from build123d import *

# Parameters (mm, degrees)
F1_DEPTH = 6.35


with BuildPart() as f1:
    # F0 (on Front) → F1 (new body, symmetric)
    with BuildSketch(Plane.XZ):
        Polygon((0, 190.5), (-1066.8, 190.5), (-1066.8, 177.8), (-1104.9, 177.8), (-1104.9, 129.54), (-1066.8, 129.54), (-1066.8, 0), (-1066.8, -129.54), (-1104.9, -129.54), (-1104.9, -177.8), (-1066.8, -177.8), (-1066.8, -190.5), (0, -190.5), (1066.8, -190.5), (1066.8, -177.8), (1104.9, -177.8), (1104.9, -129.54), (1066.8, -129.54), (1066.8, 0), (1066.8, 129.54), (1104.9, 129.54), (1104.9, 177.8), (1066.8, 177.8), (1066.8, 190.5), align=None)
    extrude(amount=F1_DEPTH, both=True)


solid = f1.part
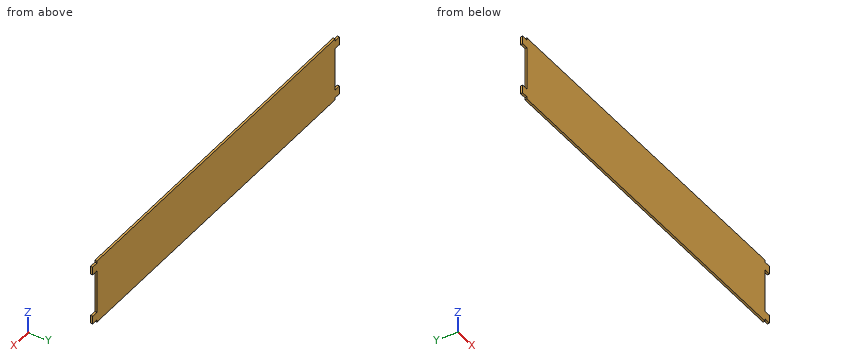
Read the model definition and answer for the solid it produces. Units are mm, in the model's axes. Give positions to 0.01 mm unless a question says otherwise; leave off trailing zeros. Loops run counter-clockwise (first coordinate to the right, second up) from the corner with the lowest first, then second, coordinate; pieces in that order, holes last. Notation, with made-up numbers: (46.25, -3.75) -> (54.25, -3.75) arc R14 cw to (54.25, 15.25) -> close; hole circle Ø7 at (65, -12). An arc over 180 degrees is marked (long way). Use a Markdown table: item, result.
Q1. Find the intervals of material crossed by line 1 along X through (y, z) = (-2.25, -79), in increasing order.
Solved:
| item | result |
|---|---|
| line 1 | x = -1066.8 to 1066.8 |
Q2. Section A-A, the plane y = 0.75 is taken. Determine the outline of the cut face in (x, z), then the cut area to 3 significant figures.
Solved:
| item | result |
|---|---|
| outline | (-1104.9, -177.8) -> (-1066.8, -177.8) -> (-1066.8, -190.5) -> (1066.8, -190.5) -> (1066.8, -177.8) -> (1104.9, -177.8) -> (1104.9, -129.54) -> (1066.8, -129.54) -> (1066.8, 129.54) -> (1104.9, 129.54) -> (1104.9, 177.8) -> (1066.8, 177.8) -> (1066.8, 190.5) -> (-1066.8, 190.5) -> (-1066.8, 177.8) -> (-1104.9, 177.8) -> (-1104.9, 129.54) -> (-1066.8, 129.54) -> (-1066.8, -129.54) -> (-1104.9, -129.54) -> close |
| area | 820,000 mm^2 |
Q3. Section B-B, the plane z = 47.5 is taken. Determine the outline of the cut face in (x, y).
Solved:
| item | result |
|---|---|
| outline | (-1066.8, -6.35) -> (1066.8, -6.35) -> (1066.8, 6.35) -> (-1066.8, 6.35) -> close |
Q4. Each of these flat-tipped pins is pushed along its axis until it touches: pin 1 (6.5 mm diameter, centred on x = 1093, y = 3, fed in from +Z); pin 2 (4 mm diameter, centred on x = 1084.5, y = -1.5, fed in from -Z); pin 3 (2 mm diameter, centred on y = -5, z = -85.5, fed in from -X). Where does it stop, or does it pass through?
Solved:
| item | result |
|---|---|
| pin 1 | stops at z = 177.8 |
| pin 2 | stops at z = -177.8 |
| pin 3 | stops at x = -1066.8 |
